from build123d import *

# Parameters (mm, degrees)
SKETCH1_R           = 7.5
BOSS_EXTRUDE1_DEPTH = 10
SKETCH2_R           = 10
BOSS_EXTRUDE2_DEPTH = 18
CHAMFER1_SIZE       = 2
CHAMFER1_SIZE2      = 11.342563639


with BuildPart() as part:
    # Sketch1 → Boss-Extrude1 (new body)
    with BuildSketch(Plane.XY):
        Circle(SKETCH1_R)
    extrude(amount=BOSS_EXTRUDE1_DEPTH)

    # Sketch2 → Boss-Extrude2 (add)
    with BuildSketch(Plane.XY.offset(10)):
        Circle(SKETCH2_R)
    extrude(amount=BOSS_EXTRUDE2_DEPTH)

    # Chamfer1
    chamfer1_edges = [part.edges().sort_by_distance(p)[0] for p in [
        (-10, 0, 28),
    ]]
    chamfer1_side = [part.faces().sort_by_distance(p)[0] for p in [
        (0, 0, 28),
    ]]
    chamfer(chamfer1_edges, length=CHAMFER1_SIZE, length2=CHAMFER1_SIZE2, reference=chamfer1_side[0])


solid = part.part
For this review, take the finished solid that the model builds, in its own axes (mm). A direction names the side the tool comes from. Give positions to 0.01 mm unless a question says otherwise; leave off trailing zeros. Loops run counter-clockwise (first coordinate to the right, second up) from the corner with the lowest first, then second, coordinate; pieces in that order, holes last.
Item 1: For line 1 along Y through (x, z) = (0, 9.75); line 2 along X through (y, z) = (-4.5, 22.25); line 3 along Y through (x, z) = (-1, 6), list the stretches that pass through material, from the lowest coordinate up.
Item 2: Take a section at A-A, the plane x = 0. State the section outline as (y, z) points, and give its area (3 significant figures).
Item 3: Take a section at D-D, the plane z = 23.25. State the section outline as (x, y) points.
Item 4: Take a section at C-C, the plane z = 10.5. State the section outline as (x, y) points.
Item 5: Tool access review of faces 1 (the flat face through (0, 0, 28)), 2 (the flat face through (4, 7, 10)): name each direction out of +Z, -Z, +X, -X, +Y, -Y from which nothing blocks a thin tool from reaching the whole face with its end or side.
Item 6: Insertion check: pin 1 (3 mm diameter, centred on y = -1, z = 18.5, fed in from -X); pin 2 (10 mm diameter, centred on x = 7, z = 14.5, fed in from +Y); pin 3 (1.5 mm diameter, centred on x = 4, y = -7.5, fed in from -Z). Each pin has a flat end and moves straight along its axis. Give the tip position at first contact, or say it passes through.
Calculated:
1. line 1: y = -7.5 to 7.5
1. line 2: x = -7.81 to 7.81
1. line 3: y = -7.43 to 7.43
2. outline: (-10, 10) - (-7.5, 10) - (-7.5, 0) - (7.5, 0) - (7.5, 10) - (10, 10) - (10, 16.66) - (8, 28) - (-8, 28) - (-10, 16.66) - close
2. area: 487 mm2
3. outline: circle Ø17.68 at (0, 0)
4. outline: circle Ø20 at (0, 0)
5. face 1: +Z, +X, -X, +Y, -Y
5. face 2: -Z
6. pin 1: stops at x = -9.91
6. pin 2: stops at y = 9.8
6. pin 3: stops at z = 10
